from build123d import *

# Parameters (mm, degrees)
F0_W     = 8.57504
F0_H     = 8.763
F0_W_2   = 8.56996
F1_DEPTH = 6.35
F2_W     = 104.775
F2_H     = 3.175
F3_DEPTH = 8.6106


with BuildPart() as f1:
    # F0 (on Top) → F1 (new body)
    with BuildSketch(Plane.XY):
        with Locations((-4.28752, 4.3815)):
            Rectangle(F0_W, F0_H)
        with BuildLine():
            Line((0, 8.763), (0, 0))
            Line((0, 0), (87.63, 0))
            Line((87.63, 0), (87.63, 8.763))
            Line((87.63, 8.763), (87.63, 18.288))
            Line((87.63, 18.288), (87.63, 50.77453))
            ThreePointArc((87.63, 50.77453), (49.462914, 57.239683), (10.752161, 57.287836))
            ThreePointArc((10.752161, 57.287836), (4.343582, 54.59828), (0, 49.172703))
            Line((0, 49.172703), (0, 18.288))
            Line((0, 18.288), (0, 8.763))
        make_face()
        with BuildLine():
            Line((78.486, 18.288), (9.144, 18.288))
            Line((9.144, 18.288), (9.144, 45.242749))
            ThreePointArc((9.144, 45.242749), (12.091924, 51.224816), (18.373285, 53.465328))
            ThreePointArc((18.373285, 53.465328), (48.594074, 52.979261), (78.486, 48.50655))
            Line((78.486, 48.50655), (78.486, 18.288))
        make_face(mode=Mode.SUBTRACT)
        with Locations((91.91498, 4.3815)):
            Rectangle(F0_W_2, F0_H)
    extrude(amount=F1_DEPTH)

    # F2 (on face) → F3 (cut)
    with BuildSketch(Plane.XZ):
        with Locations((43.81246, 3.175)):
            Rectangle(F2_W, F2_H)
    extrude(amount=-F3_DEPTH, mode=Mode.SUBTRACT)


solid = f1.part
Check sheet for the modelled part. Datum: model origin and axes. Units: mm. A direction names the side the tool comes from. Round coordinates to 2 decimals unless told otherwise and drop trailing zeros. Write each loop counter-clockwise with the first axis right and the second up, starting at its lowest first coordinate (ties: lowest second). Pieces come first, ordered by that corner, then holes. Notation, with made-up numbers: (88.5, 88.5) -> (102.5, 88.5) arc R22 cw to (102.5, 112.5) -> close; hole circle Ø9 at (62.25, 32.25). An arc over 180 degrees is marked (long way). Answer as CSV lines item,"result". Start each with the question number.
1) Section check C-C on z = 3.75. Enter the section's corners in (x, y).
2) Section check A-A on y = 32. Enter the section's corners in (x, z).
3) Material ranges on line 1 (X direction, y = 28, z = 3.75); line 2 (X direction, y = 10.5, z = 3.5); line 3 (Z direction, x = 15.5, y = 7.5), recorded low to high. Write a range as from..to.
4) Section check D-D on x = 40. Enter the section's corners in (y, z).
5) Tool access check on faces 1 (the cylindrical face through (48.172, 53.014, 3.131)), 2 (the flat face through (87.63, 29, 3)), 3 (the flat face through (43, 4, 1.588)), 4 (the flat face through (0, 29, 3)). Record the directions out of +Z, -Z, +X, -X, +Y, -Y that give a thin tool (end or side, any length) a straight path to the whole face; none if there is none.
6) Release check for a two-part mould opening along Y. For faces 5 (the cylindrical face through (50.004, 57.193, 3.131)), 6 (the flat face through (-8.575, 4, 1)), 7 (the flat face through (78.486, 34, 3)) record: pulls with the +Y half, pulls with the -Y half, needs draft (parallel to the pull), parting line crosses it, or undercut.
7) Go/stop test with flat-tipped pins: P1, Ø1, axis at x = 53.5, z = 3.5, coming from the -Y side; P2, Ø3, axis at y = 33.5, z = 2.5, coming from the -X side; P3, Ø1.9, axis at x = -5, z = 4.5, coming from the +Y side. Record where each tip stops, or that it passes through.
8) Section check B-B on x = 54. Enter the section's corners in (y, z).
Found:
1,outline,"(-8.58, 8.61) -> (96.2, 8.61) -> (96.2, 8.76) -> (87.63, 8.76) -> (87.63, 50.77) arc R232.69 ccw to (10.75, 57.29) arc R14.09 ccw to (0, 49.17) -> (0, 8.76) -> (-8.58, 8.76) -> close; hole (9.14, 18.29) -> (78.49, 18.29) -> (78.49, 48.51) arc R228.37 ccw to (18.37, 53.47) arc R8.88 ccw to (9.14, 45.24) -> close"
2,outline,"(0, 0) -> (9.14, 0) -> (9.14, 6.35) -> (0, 6.35) -> close; (78.49, 0) -> (87.63, 0) -> (87.63, 6.35) -> (78.49, 6.35) -> close"
3,line 1,"x = 0..9.14, 78.49..87.63"
3,line 2,"x = 0..87.63"
3,line 3,"z = 0..1.59, 4.76..6.35"
4,outline,"(0, 0) -> (18.29, 0) -> (18.29, 6.35) -> (0, 6.35) -> (0, 4.76) -> (8.61, 4.76) -> (8.61, 1.59) -> (0, 1.59) -> close; (53.53, 0) -> (57.85, 0) -> (57.85, 6.35) -> (53.53, 6.35) -> close"
5,face 1,"+Z, -Z"
5,face 2,"+Z, -Z, +X, +Y"
5,face 3,"+X, -X, -Y"
5,face 4,"+Z, -Z, -X, +Y"
6,face 5,"pulls with the +Y half"
6,face 6,"needs draft"
6,face 7,"undercut"
7,P1,"stops at y = 8.61"
7,P2,"stops at x = 0"
7,P3,"stops at y = 8.76"
8,outline,"(0, 0) -> (18.29, 0) -> (18.29, 6.35) -> (0, 6.35) -> (0, 4.76) -> (8.61, 4.76) -> (8.61, 1.59) -> (0, 1.59) -> close; (52.47, 0) -> (56.81, 0) -> (56.81, 6.35) -> (52.47, 6.35) -> close"
